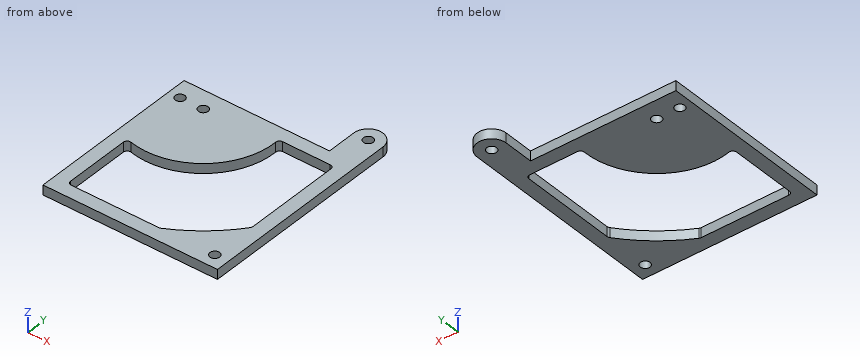
```python
from build123d import *

# Parameters (mm, degrees)
SKETCH1_R           = 3.175
BOSS_EXTRUDE1_DEPTH = 3.175


with BuildPart() as part:
    # Sketch1 → Boss-Extrude1 (new, symmetric)
    with BuildSketch(Plane.XY):
        with BuildLine():
            Line((-57.15, -57.15), (57.15, -57.15))
            Line((57.15, -57.15), (57.15, 76.835))
            ThreePointArc((57.15, 76.835), (47.625, 86.36), (38.1, 76.835))
            Line((38.1, 76.835), (38.1, 57.15))
            Line((38.1, 57.15), (-57.15, 57.15))
            Line((-57.15, 57.15), (-57.15, -57.15))
        make_face()
        with Locations((-49.53, 44.45)):
            Circle(SKETCH1_R, mode=Mode.SUBTRACT)
        with Locations((-34.29, 44.45)):
            Circle(SKETCH1_R, mode=Mode.SUBTRACT)
        with Locations((48.26, -48.25058611)):
            Circle(SKETCH1_R, mode=Mode.SUBTRACT)
        with Locations((47.625, 76.835)):
            Circle(SKETCH1_R, mode=Mode.SUBTRACT)
        with BuildLine():
            Line((-45.77152391, -48.25058611), (11.571822448, -48.25058611))
            ThreePointArc((11.571822448, -48.25058611), (12.151642643, -48.182093861), (12.69954516, -47.980387445))
            ThreePointArc((12.69954516, -47.980387445), (31.830233088, -35.421826409), (47.740202739, -18.972706629))
            ThreePointArc((47.740202739, -18.972706629), (48.126468012, -18.254805898), (48.26, -17.450597264))
            Line((48.26, -17.450597264), (48.26, 45.77152391))
            ThreePointArc((48.26, 45.77152391), (47.531142228, 47.531142228), (45.77152391, 48.26))
            Line((45.77152391, 48.26), (14.585930721, 48.26))
            ThreePointArc((14.585930721, 48.26), (12.802691065, 47.50719945), (12.09836376, 45.704264235))
            ThreePointArc((12.09836376, 45.704264235), (-5.096432418, 8.378001401), (-45.187165534, -0.657707262))
            ThreePointArc((-45.187165534, -0.657707262), (-47.310736599, -1.121263606), (-48.26, -3.076599268))
            Line((-48.26, -3.076599268), (-48.26, -45.76211002))
            ThreePointArc((-48.26, -45.76211002), (-47.531142228, -47.521728338), (-45.77152391, -48.25058611))
        make_face(mode=Mode.SUBTRACT)
    extrude(amount=BOSS_EXTRUDE1_DEPTH, both=True)


solid = part.part
```
The model under review builds one solid part; all positions refer to its coordinate system, in mm. Round coordinates to 2 decimals unless told otherwise and drop trailing zeros. Write each loop counter-clockwise with the first axis right and the second up, starting at its lowest first coordinate (ties: lowest second). Pieces come first, ordered by that corner, then holes. Notation, with made-up numbers: (21, 43.5) - (69, 43.5) arc R15 cw to (69, 67.5) - close; hole circle Ø3 at (-7, 46.25). An arc over 180 degrees is marked (long way). Answer as CSV lines item,"result". Start each with the question number.
(1) We need section A-A on y = -15. State the section outline as (x, z) points (3 decimals).
(2) For pin 1 Ø5.5 at (x, y) = (-34.29, 44.45) entering from -Z; pin 2 Ø7.5 at (x, y) = (48.26, -48.25) entering from +Z (3 decimals); pin 3 Ø1.9 at (x, z) = (-3.5, 1.5) entering from +Y, all flat-tipped, find the tip position at first contact; note any pin that passes through.
(3) We need section C-C on z = -1.75. State the section outline as (x, y) points (3 decimals), plus the area to 3 significant figures.
(4) To check wall thickness, follow line 1 (Y direction, x = -34.29, z = -0.75) (3 decimals); line 2 (X direction, y = -17.5, z = 0); line 3 (Y direction, x = -43, z = 1.5). State the ranges of each line that lie inside material, in increasing order.
(5) We need section D-D on x = 32.5. State the section outline as (y, z) points (3 decimals).
(6) We need section B-B on x = -34.29. State the section outline as (y, z) points (3 decimals), plus the area to 3 significant figures.
Worked answers:
1,outline,"(-57.15, -3.175) - (-48.26, -3.175) - (-48.26, 3.175) - (-57.15, 3.175) - close; (48.26, -3.175) - (57.15, -3.175) - (57.15, 3.175) - (48.26, 3.175) - close"
2,pin 1,"through"
2,pin 2,"z = 3.175"
2,pin 3,"y = 57.15"
3,outline,"(-57.15, -57.15) - (57.15, -57.15) - (57.15, 76.835) arc R9.525 ccw to (38.1, 76.835) - (38.1, 57.15) - (-57.15, 57.15) - close; hole circle Ø6.35 at (-49.53, 44.45); hole (-48.26, -45.762) arc R2.488 ccw to (-45.772, -48.251) - (11.572, -48.251) arc R2.488 ccw to (12.7, -47.98) arc R103.689 ccw to (47.74, -18.973) arc R2.488 ccw to (48.26, -17.451) - (48.26, 45.772) arc R2.488 ccw to (45.772, 48.26) - (14.586, 48.26) arc R2.488 ccw to (12.098, 45.704) arc R46.405 cw to (-45.187, -0.658) arc R2.488 ccw to (-48.26, -3.077) - close; hole circle Ø6.35 at (-34.29, 44.45); hole circle Ø6.35 at (47.625, 76.835); hole circle Ø6.35 at (48.26, -48.251)"
3,area,"7,160 mm²"
4,line 1,"-57.15 to -48.251, -1.955 to 41.275, 47.625 to 57.15"
4,line 2,"-57.15 to -48.26, 48.26 to 57.15"
4,line 3,"-57.15 to -48.25, -1.13 to 57.15"
5,outline,"(-57.15, -3.175) - (-34.863, -3.175) - (-34.863, 3.175) - (-57.15, 3.175) - close; (48.26, -3.175) - (57.15, -3.175) - (57.15, 3.175) - (48.26, 3.175) - close"
6,outline,"(-57.15, -3.175) - (-48.251, -3.175) - (-48.251, 3.175) - (-57.15, 3.175) - close; (-1.955, -3.175) - (41.275, -3.175) - (41.275, 3.175) - (-1.955, 3.175) - close; (47.625, -3.175) - (57.15, -3.175) - (57.15, 3.175) - (47.625, 3.175) - close"
6,area,"392 mm²"
